Source: CAD feature listing. Evaluate the final solid. Frame: model axes, mm. A direction names the side the tool comes from. Coordinates: 2 decimals unless noted, no trailing zeros. Order: outer loops, then holes, each group sorted by start corner. A loop starts at its lowest first (then second) coordinate and runs counter-clockwise, first axis right, second up.
```python
from build123d import *

# Parameters (mm, degrees)
F0_R     = 1.5
F1_DEPTH = 3
F2_R     = 10
F3_SIZE  = 10


with BuildPart() as f1:
    # F0 (on Top) → F1 (new body)
    with BuildSketch(Plane.XY):
        Polygon((-35.355339, 18.384776), (-16.970563, 0), (-35.355339, -18.384776), (-18.384776, -35.355339), (0, -16.970563), (18.384776, -35.355339), (35.355339, -18.384776), (16.970563, 0), (35.355339, 18.384776), (18.384776, 35.355339), (0, 16.970563), (-18.384776, 35.355339), align=None)
        with Locations((-16.793786, -25.632621)):
            Circle(F0_R, mode=Mode.SUBTRACT)
        with Locations((-9.722718, -18.561553)):
            Circle(F0_R, mode=Mode.SUBTRACT)
        with Locations((-25.632621, -16.793786)):
            Circle(F0_R, mode=Mode.SUBTRACT)
        with Locations((-18.561553, -9.722718)):
            Circle(F0_R, mode=Mode.SUBTRACT)
        with Locations((16.793786, -25.632621)):
            Circle(F0_R, mode=Mode.SUBTRACT)
        with Locations((9.722718, -18.561553)):
            Circle(F0_R, mode=Mode.SUBTRACT)
        with Locations((25.632621, -16.793786)):
            Circle(F0_R, mode=Mode.SUBTRACT)
        with Locations((18.561553, -9.722718)):
            Circle(F0_R, mode=Mode.SUBTRACT)
        with Locations((-18.561553, 9.722718)):
            Circle(F0_R, mode=Mode.SUBTRACT)
        with Locations((-25.632621, 16.793786)):
            Circle(F0_R, mode=Mode.SUBTRACT)
        with Locations((-9.722718, 18.561553)):
            Circle(F0_R, mode=Mode.SUBTRACT)
        with Locations((-16.793786, 25.632621)):
            Circle(F0_R, mode=Mode.SUBTRACT)
        with Locations((18.561553, 9.722718)):
            Circle(F0_R, mode=Mode.SUBTRACT)
        with Locations((25.632621, 16.793786)):
            Circle(F0_R, mode=Mode.SUBTRACT)
        with Locations((9.722718, 18.561553)):
            Circle(F0_R, mode=Mode.SUBTRACT)
        with Locations((16.793786, 25.632621)):
            Circle(F0_R, mode=Mode.SUBTRACT)
    extrude(amount=F1_DEPTH)

    # F2
    f2_edges = [f1.edges().sort_by_distance(p)[0] for p in [
        (-16.970563, 0, 1.5),
        (16.970563, 0, 1.5),
    ]]
    fillet(f2_edges, radius=F2_R)

    # F3
    f3_edges = [f1.edges().sort_by_distance(p)[0] for p in [
        (0, -16.970563, 1.5),
        (0, 16.970563, 1.5),
    ]]
    chamfer(f3_edges, length=F3_SIZE)


solid = f1.part
```
1. Section query B-B on z = 0.6. Count the separate pieces of the cut face and the enclosed holes in it, plus the area to 3 significant figures.
Findings:
separate pieces: 1
enclosed holes: 16
area: 3,100 mm2
2. Ray query, line 1 (X direction, y = 10, z = 0.95); line 2 (Y direction, x = -17, z = 2.75); line 3 (Y direction, x = -9, z = 1.3). Return the intervals inside material, ascending.
Findings:
line 1: x = -26.97 to -20.04, -17.09 to 17.09, 20.04 to 26.97
line 2: y = -33.97 to -27.12, -24.15 to 24.15, 27.12 to 33.97
line 3: y = -25.97 to -19.88, -17.25 to 17.25, 19.88 to 25.97
3. Pin query (flat end, axial travel): P1, Ø0.9, axis at x = -3.5, z = 1, coming from the +Y side; P2, Ø1.5, axis at y = -14, z = 2.5, coming from the +X side; P3, Ø2.5, axis at x = -25.63, y = -16.79, coming from the -Z side; P4, Ø4, axis at x = 9.72, y = 18.56, coming from the -Z side. Return the tip coordinate at first contact, or that it passes through.
Findings:
P1: stops at y = 24.04
P2: stops at x = 31.72
P3: passes through
P4: stops at z = 0
4. Section query C-C on x = -26. Return loops of the section in (y, z).
Findings:
outline: (-27.74, 0) - (-18.25, 0) - (-18.25, 3) - (-27.74, 3) - close; (-15.34, 0) - (-9.03, 0) - (-9.03, 3) - (-15.34, 3) - close; (9.03, 0) - (15.34, 0) - (15.34, 3) - (9.03, 3) - close; (18.25, 0) - (27.74, 0) - (27.74, 3) - (18.25, 3) - close
5. Draft query along Y for faces 1 (the face through (18.225, 26.083, 1.479)), 2 (the face through (12.65, -29.62, 1.48)), 3 (the face through (26.99, 26.75, 1.48)), 4 (the face through (21.113, 0.11, 1.521)). Return one class per face: released by +Y, released by -Y, zero draft, split by the parting line, or undercut.
Findings:
face 1: undercut
face 2: released by -Y
face 3: released by +Y
face 4: undercut
6. Access query for faces 5 (the face through (29.62, 12.65, 1.48)), 6 (the face through (-29.62, -12.65, 1.48)), 7 (the face through (0, 24.042, 1)), 8 (the face through (-16.99, 27.12, 1.48)). Directions: +Z, -Z, +X, -X, +Y, -Y. A direction counts if a zero-diameter tool reaches every point of the face in a straight line with its end or side. Return the directions, or none.
Findings:
face 5: +Z, -Z, +X
face 6: +Z, -Z, -X
face 7: +Z, -Z, +Y
face 8: +Z, -Z
7. Section query D-D on x = -9.5. Return loops of the section in (y, z), plus the area to 3 significant figures.
Findings:
outline: (-26.47, 0) - (-20.04, 0) - (-20.04, 3) - (-26.47, 3) - close; (-17.08, 0) - (17.08, 0) - (17.08, 3) - (-17.08, 3) - close; (20.04, 0) - (26.47, 0) - (26.47, 3) - (20.04, 3) - close
area: 141 mm2
8. Section query A-A on x = 29. Return loops of the section in (y, z).
Findings:
outline: (-24.74, 0) - (-12.03, 0) - (-12.03, 3) - (-24.74, 3) - close; (12.03, 0) - (24.74, 0) - (24.74, 3) - (12.03, 3) - close
